Autodesk Inventor part; units mm, degrees
ref_plane "YZ Plane" through (0, 0, 0) normal (1, 0, 0) x (0, 1, 0)
ref_plane "XZ Plane" through (0, 0, 0) normal (0, 1, 0) x (-1, 0, 0)
ref_plane "XY Plane" through (0, 0, 0) normal (0, 0, 1) x (1, 0, 0)
sketch "Sketch1" plane through (0, 0, 0) normal (0, 0, 1) x (1, 0, 0)
  line L0 (-49.634624, 71.104228) -> (-18.657482, 93.113696)
  circle A0 centre (-49.634624, 71.104228) radius 5
  circle A1 centre (-18.657482, 93.113696) radius 5
  circle A2 centre (-49.634624, 71.104228) radius 3.075
  circle A3 centre (-18.657482, 93.113696) radius 3.075
  line L1 (-49.634624, 71.104228) -> (-18.657482, 93.113696) construction
  line L2 (-48.62103, 69.677649) -> (-17.643888, 91.687117)
  line L3 (-19.671076, 94.540275) -> (-50.648218, 72.530807)
  arc A4 (-50.648218, 72.530807) -> (-48.62103, 69.677649) centre (-49.634624, 71.104228) ccw
  arc A5 (-17.643888, 91.687117) -> (-19.671076, 94.540275) centre (-18.657482, 93.113696) ccw
  line L4 (-18.657482, 93.113696) -> (-2.353723, 104.697626) construction
  line L5 (-17.643888, 91.687117) -> (-1.340129, 103.271047)
  line L6 (-3.367317, 106.124205) -> (-19.671076, 94.540275)
  arc A6 (-19.671076, 94.540275) -> (-17.643888, 91.687117) centre (-18.657482, 93.113696) ccw
  arc A7 (-1.340129, 103.271047) -> (-3.367317, 106.124205) centre (-2.353723, 104.697626) ccw
  line L7 (-2.353723, 104.697626) -> (-3.367317, 106.124205)
  line L8 (-2.353723, 104.697626) -> (-1.340129, 103.271047)
  point P0 (0, 0)
  point P1 (-34.146053, 82.108962)
  point P2 (-10.505602, 98.905661)
  point P3 (-44.802894, 72.39046)
  point P4 (-21.462023, 88.974306)
  point P5 (-13.825752, 94.399928)
  point P6 (-15.85294, 97.253085)
  point P7 (-23.489211, 91.827464)
  point P8 (-46.830082, 75.243618)
  dimension "d0" = 10
  dimension "d1" = 10
  dimension "d2" = 6.15
  dimension "d3" = 6.15
  dimension "d4" = 3.5
  dimension "d5" = 20
  dimension "d6" = 3.5
sketch "Sketch1 outline for Extrusion1" plane through (0, 0, 0) normal (0, 0, 1) x (1, 0, 0)
  line L0 (-44.802894, 72.39046) -> (-21.462023, 88.974306)
  arc A0 (-46.830082, 75.243618) -> (-44.802894, 72.39046) centre (-49.634624, 71.104228) ccw
  arc A1 (-21.462023, 88.974306) -> (-13.825752, 94.399928) centre (-18.657482, 93.113696) ccw
  line L1 (-23.489211, 91.827464) -> (-46.830082, 75.243618)
  line L2 (-13.825752, 94.399928) -> (-1.340129, 103.271047)
  arc A2 (-15.85294, 97.253085) -> (-23.489211, 91.827464) centre (-18.657482, 93.113696) ccw
  line L3 (-1.340129, 103.271047) -> (-2.353723, 104.697626)
  line L4 (-3.367317, 106.124205) -> (-15.85294, 97.253085)
  line L5 (-2.353723, 104.697626) -> (-3.367317, 106.124205)
  circle A3 centre (-49.634624, 71.104228) radius 3.075
  circle A4 centre (-18.657482, 93.113696) radius 3.075
extrude "Extrusion1" add sketch "Sketch1 outline for Extrusion1" along normal mid plane 7
sketch "Sketch2" plane through (-1.340129, 103.271047, -3.5) normal (0.5791965, -0.8151879, 0) x (0.8151879, 0.5791965, 0)
  line L0 (0, 0) -> (0, 7)
  line L1 (-15.316252, 7) -> (0, 7)
  line L2 (-15.316252, 0) -> (-15.316252, 7)
  line L3 (0, 0) -> (-15.316252, 0)
  line L4 (0, 0) -> (0, 7)
  line L5 (0, 3.5) -> (-8, 3.5)
  line L6 (-8, 3.5) -> (-3, 3.5)
  circle A0 centre (-3, 3.5) radius 1
  line L7 (-8, 3.5) -> (-10, 3.5)
  circle A1 centre (-10, 3.5) radius 1
  point P0 (-58.721774, 3.5)
  dimension "d9" = 8
  dimension "d10" = 5
  dimension "d11" = 2
  dimension "d12" = 2
  dimension "d13" = 2
sketch "Sketch2 outline for Extrusion2" plane through (-1.340129, 103.271047, -3.5) normal (0.5791965, -0.8151879, 0) x (0.8151879, 0.5791965, 0)
  circle A0 centre (-3, 3.5) radius 1
  circle A1 centre (-10, 3.5) radius 1
extrude "Extrusion2" cut sketch "Sketch2 outline for Extrusion2" against normal blind 5
fillet "Fillet1" radius 2 6 edges at (-46.8301, 75.2436, 0) (-44.8029, 72.3905, 0) (-21.462, 88.9743, 0) (-13.8258, 94.3999, 0) (-15.8529, 97.2531, 0) (-23.4892, 91.8275, 0)
chamfer "Chamfer1" distance 2 angle 45 2 edges at (-2.3537, 104.6976, 3.5) (-2.3537, 104.6976, -3.5)
properties part number "leg_link_1"
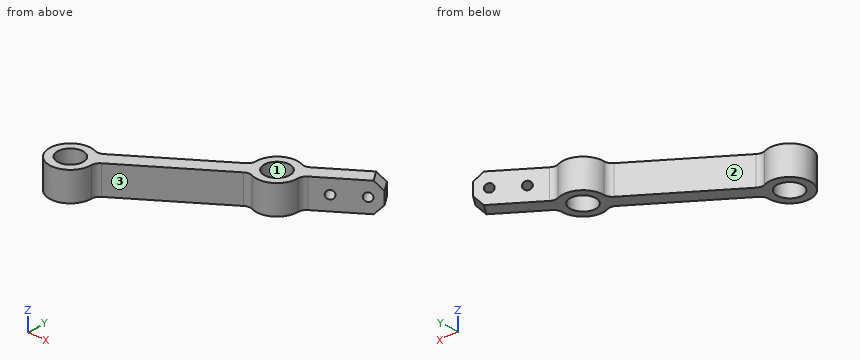
Source: CAD feature listing. Evaluate the final solid. Frame: model axes, mm. Face numbers are marked on the shaded views. Coordinates: 2 decimals unless noted, no trailing zeros. Loops run counter-clockwise (first coordinate to the right, second up) from the corner with the lowest first, then second, coordinate; pieces in that order, holes last. Notation, with made-up numbers: M 69,-29.75 L 118,-29.75 A13 cw 118,-8.75 Z; hole C 89,58.5 d3. An arc over 180 degrees is marked long. Use a Markdown table: item, result. Add a question column.
Q1. Draft query along Y for the marked faces 1, 2 and 3. Return one class per face: pulls with the +Y half, pulls with the -Y half, needs draft (parallel to the pull), parting line crosses it, or undercut.
Q2. Section query D-D, the plane z = -2.75. Return loops of the section in (x, y) (3 decimals), and give its area (3 significant figures).
Q3. Section query B-B, the plane z = 2.5. State how many separate pieces and enclosed holes the cut face has, and give its area (3 significant figures).
Q4. Section query C-C, the plane y = 69.5. Return loops of the section in (x, z).
Q5. Material intervals for L1, parallel to X at y = 71, z = 2.25; L2, parallel to X at y = 69.5, z = -3; L3, parallel to Y at x = -20, z = 0.25, sorted ascending.
Q6. First-contact query: pin 1 (2 mm diameter, centred on y = 100, z = -1, fed in from +X); pin 2 (3.5 mm diameter, centred on x = -18.66, y = 93.11, fed in from +Z); pin 3 (1.5 mm diameter, centred on y = 82.5, z = -3, fed in from +X). Flat tips, straight axial feed; report the tip coordinate or a pass-through.
Q7. Section query A-A, the plane y = 94. Return loops of the section in (x, z), and give its area (3 significant figures).
Result:
| question | item | result |
|---|---|---|
| 1 | face 1 | undercut |
| 1 | face 2 | pulls with the +Y half |
| 1 | face 3 | pulls with the -Y half |
| 2 | outline | M -47.744,75.733 A5 ccw long -44.641,71.366 A2 cw -43.803,73.101 L -22.462,88.264 A2 cw -20.548,88.485 A5 ccw -13.664,93.376 A2 cw -12.825,95.111 L -2.359,102.547 L -4.386,105.4 L -14.853,97.964 A2 cw -16.767,97.743 A5 ccw -23.651,92.852 A2 cw -24.489,91.117 L -45.83,75.954 A2 cw Z; hole C -49.635,71.104 d6.15; hole C -18.657,93.114 d6.15 |
| 2 | area | 246 mm2 |
| 3 | separate pieces | 1 |
| 3 | enclosed holes | 2 |
| 3 | area | 247 mm2 |
| 4 | outline | M -54.37,-3.5 L -52.26,-3.5 L -52.26,3.5 L -54.37,3.5 Z; M -47.01,-3.5 L -44.9,-3.5 L -44.9,3.5 L -47.01,3.5 Z |
| 5 | L1 | x = -54.63 to -52.71, -46.56 to -44.64 |
| 5 | L2 | x = -54.37 to -52.26, -47.01 to -44.9 |
| 5 | L3 | y = 88.3 to 90.35, 95.88 to 97.93 |
| 6 | pin 1 | stops at x = -4.54 |
| 6 | pin 2 | passes through |
| 6 | pin 3 | stops at x = -29.52 |
| 7 | outline | M -23.58,-3.5 L -21.6,-3.5 L -21.6,3.5 L -23.58,3.5 Z; M -15.71,-3.5 L -13.6,-3.5 L -13.6,3.5 L -15.71,3.5 Z |
| 7 | area | 28.6 mm2 |
